```python
from build123d import *

# Parameters (mm, degrees)
SALIENTE_EXTRUIR1_DEPTH      = 35
SALIENTE_EXTRUIR1_DEPTH_BACK = 35
CORTAR_EXTRUIR1_DEPTH        = 3
CROQUIS4_R                   = 8
CORTAR_EXTRUIR2_DEPTH        = 3
CROQUIS5_R                   = 2.5
CORTAR_EXTRUIR3_DEPTH        = 10
CROQUIS6_W                   = 6
CROQUIS6_H                   = 10
CORTAR_EXTRUIR5_DEPTH        = 10
CROQUIS7_W                   = 2
CROQUIS7_H                   = 2
CORTAR_EXTRUIR6_DEPTH        = 5
CROQUIS8_R                   = 1
CORTAR_EXTRUIR7_DEPTH        = 2
CROQUIS9_W                   = 6
CROQUIS9_H                   = 10
CORTAR_EXTRUIR8_DEPTH        = 12
CORTAR_EXTRUIR9_DEPTH        = 5
CORTAR_EXTRUIR9_DEPTH_BACK   = 5
CROQUIS10_R                  = 1
CORTAR_EXTRUIR10_DEPTH       = 5
CORTAR_EXTRUIR10_DEPTH_BACK  = 5
CORTAR_EXTRUIR11_DEPTH       = 3
CORTAR_EXTRUIR11_DEPTH_BACK  = 3
CROQUIS15_R                  = 2.5
CORTAR_EXTRUIR12_DEPTH       = 15
CROQUIS14_W                  = 2
CROQUIS14_H                  = 10
CORTAR_EXTRUIR13_DEPTH       = 10


with BuildPart() as part:
    # Croquis1 → Saliente-Extruir1 (new, two sides: drawn at the far end of the back side and taken through both)
    with BuildSketch(Plane.XY.offset(-SALIENTE_EXTRUIR1_DEPTH_BACK)):
        with BuildLine():
            Line((-15, 0), (15, 0))
            ThreePointArc((15, 0), (0, -15), (-15, 0))
        make_face()
    extrude(amount=SALIENTE_EXTRUIR1_DEPTH + SALIENTE_EXTRUIR1_DEPTH_BACK)

    # Croquis3 → Cortar-Extruir1 (cut)
    with BuildSketch(Plane(origin=(0, 0, 0), x_dir=(1, 0, 0), z_dir=(0, 1, 0))):
        with BuildLine():
            Line((-8, 25), (-12.284525276, 15.598253186))
            ThreePointArc((-12.284525276, 15.598253186), (0, -3.5), (12.284525276, 15.598253186))
            Line((12.284525276, 15.598253186), (8, 25))
            ThreePointArc((8, 25), (13, 30), (8, 35))
            Line((8, 35), (-8, 35))
            ThreePointArc((-8, 35), (-13, 30), (-8, 25))
        make_face()
    extrude(amount=-CORTAR_EXTRUIR1_DEPTH, mode=Mode.SUBTRACT)

    # Croquis4 → Cortar-Extruir2 (cut)
    with BuildSketch(Plane(origin=(0, -3, 0), x_dir=(1, 0, 0), z_dir=(0, 1, 0))):
        with Locations(Location((0, 10, 0), (0, 0, 270))):
            Circle(CROQUIS4_R)
    extrude(amount=-CORTAR_EXTRUIR2_DEPTH, mode=Mode.SUBTRACT)

    # Croquis5 → Cortar-Extruir3 (cut)
    with BuildSketch(Plane(origin=(0, -6, 0), x_dir=(1, 0, 0), z_dir=(0, 1, 0))):
        with Locations(Location((0, 10, 0), (0, 0, 270))):
            Circle(CROQUIS5_R)
    extrude(amount=-CORTAR_EXTRUIR3_DEPTH, mode=Mode.SUBTRACT)

    # Croquis6 → Cortar-Extruir5 (cut)
    with BuildSketch(Plane(origin=(0, -3, 0), x_dir=(1, 0, 0), z_dir=(0, 1, 0))):
        with Locations((0, 30)):
            Rectangle(CROQUIS6_W, CROQUIS6_H)
    extrude(amount=-CORTAR_EXTRUIR5_DEPTH, mode=Mode.SUBTRACT)

    # Croquis7 → Cortar-Extruir6 (cut)
    with BuildSketch(Plane(origin=(0, -3, 0), x_dir=(1, 0, 0), z_dir=(0, 1, 0))):
        with Locations((-4, 30)):
            Rectangle(CROQUIS7_W, CROQUIS7_H)
        with Locations((4, 30)):
            Rectangle(CROQUIS7_W, CROQUIS7_H)
    extrude(amount=-CORTAR_EXTRUIR6_DEPTH, mode=Mode.SUBTRACT)

    # Croquis8 → Cortar-Extruir7 (cut)
    with BuildSketch(Plane(origin=(0, -3, 0), x_dir=(1, 0, 0), z_dir=(0, 1, 0))):
        with Locations(Location((-8, 30, 0), (0, 0, 270))):
            Circle(CROQUIS8_R)
        with Locations(Location((8, 30, 0), (0, 0, 270))):
            Circle(CROQUIS8_R)
    extrude(amount=-CORTAR_EXTRUIR7_DEPTH, mode=Mode.SUBTRACT)

    # Croquis9 → Cortar-Extruir8 (cut)
    with BuildSketch(Plane(origin=(0, -3, 0), x_dir=(1, 0, 0), z_dir=(0, 1, 0))):
        Rectangle(CROQUIS9_W, CROQUIS9_H)
    extrude(amount=-CORTAR_EXTRUIR8_DEPTH, mode=Mode.SUBTRACT)

    # Croquis10 → Cortar-Extruir9 (cut, two sides: drawn at the far end of the back side and taken through both)
    with BuildSketch(Plane(origin=(0, 0, 0), x_dir=(0, 0, -1), z_dir=(1, 0, 0)).offset(-CORTAR_EXTRUIR9_DEPTH_BACK)):
        with Locations((30, -8)):
            Circle(CROQUIS10_R)
    extrude(amount=CORTAR_EXTRUIR9_DEPTH + CORTAR_EXTRUIR9_DEPTH_BACK, mode=Mode.SUBTRACT)

    # Croquis11 → Cortar-Extruir10 (cut, two sides: drawn at the far end of the back side and taken through both)
    with BuildSketch(Plane(origin=(0, 0, 0), x_dir=(0, 0, -1), z_dir=(1, 0, 0)).offset(-CORTAR_EXTRUIR10_DEPTH_BACK)):
        with BuildLine():
            Line((-6, -15), (6, -15))
            Line((6, -15), (6, -14))
            Line((6, -14), (1, -14))
            Line((1, -14), (1, -8))
            ThreePointArc((1, -8), (0, -7), (-1, -8))
            Line((-1, -8), (-1, -14))
            Line((-1, -14), (-6, -14))
            Line((-6, -14), (-6, -15))
        make_face()
    extrude(amount=CORTAR_EXTRUIR10_DEPTH + CORTAR_EXTRUIR10_DEPTH_BACK, mode=Mode.SUBTRACT)

    # Croquis12 → Cortar-Extruir11 (cut, two sides: drawn at the far end of the back side and taken through both)
    with BuildSketch(Plane(origin=(0, 0, 0), x_dir=(0, 0, -1), z_dir=(1, 0, 0)).offset(-CORTAR_EXTRUIR11_DEPTH_BACK)):
        with BuildLine():
            Line((-3, -13), (-21.658767316, -9.861464952))
            ThreePointArc((-21.658767316, -9.861464952), (-27.635040051, -6.458030924), (-30, 0))
            Line((-30, 0), (-3, 0))
            Line((-3, 0), (-3, -13))
        make_face()
        Polygon((25, -8), (25, -3), (4, -3), (4, -13), align=None)
    extrude(amount=CORTAR_EXTRUIR11_DEPTH + CORTAR_EXTRUIR11_DEPTH_BACK, mode=Mode.SUBTRACT)

    # Croquis15 → Cortar-Extruir12 (cut)
    with BuildSketch(Plane(origin=(0, 0, 0), x_dir=(0, 0, -1), z_dir=(1, 0, 0))):
        with Locations((-20, 0)):
            Circle(CROQUIS15_R)
    extrude(amount=-CORTAR_EXTRUIR12_DEPTH, mode=Mode.SUBTRACT)

    # Croquis14 → Cortar-Extruir13 (cut)
    with BuildSketch(Plane(origin=(0, 0, 0), x_dir=(1, 0, 0), z_dir=(0, 1, 0))):
        with Locations((4, -20)):
            Rectangle(CROQUIS14_W, CROQUIS14_H)
        with Locations((-4, -20)):
            Rectangle(CROQUIS14_W, CROQUIS14_H)
    extrude(amount=-CORTAR_EXTRUIR13_DEPTH, mode=Mode.SUBTRACT)


solid = part.part
```
The model under review builds one solid part; all positions refer to its coordinate system, in mm. A direction names the side the tool comes from. Round coordinates to 2 decimals unless told otherwise and drop trailing zeros. Order: outer loops, then holes, each group sorted by start corner. A loop starts at its lowest first (then second) coordinate and runs counter-clockwise, first axis right, second up.
Item 1: Machinability: for faces 1 (the flat face through (-5, -11, 0)), 2 (the cylindrical face through (-9.9, -2.5, 20.1)), 3 (the flat face through (-5, -6, -10)), which of the approach directions +Z, -Z, +X, -X, +Y, -Y give a long, thin tool a straight path to every point of the face, cutting with its end or side? Answer none if there is none.
Working result:
face 1: -Y
face 2: -X, +Y
face 3: +Y
Item 2: Add section B-B, the plane x = -11.5. State the section outline as (y, z) points.
Working result:
outline: (-9.63, -35) - (0, -35) - (0, -33.57) - (-3, -33.57) - (-3, -26.43) - (0, -26.43) - (0, -17.32) - (-3, -17.32) - (-3, -2.93) - (0, -2.93) - (0, 17.5) arc R2.5 cw to (0, 22.5) - (0, 35) - (-9.63, 35) - close
Item 3: Draft analysis for pull direction Z (two halves, no side actions). For faces 4 (the cylindrical face through (12.024, -1.479, -3.862)), 5 (the flat face through (5, 0, 13)), state which applies: released by +Z, released by -Z, zero draft, split by the parting line, or undercut.
Working result:
face 4: undercut
face 5: zero draft
Item 4: To check wall thickness, follow probe 1 along Z at (x, y) = (0, -13.25); probe 2 along Z at (x, y) = (0, -14.05); probe 3 along X at (y, z) = (-3.8, -30). State the ranges of each line that lie inside material, in increasing order.
Working result:
probe 1: z = -35 to -12.5, -7.5 to -5, 5 to 35
probe 2: z = -35 to -12.5, -7.5 to -6, 6 to 35
probe 3: x = -14.51 to -9, -7 to -5, 5 to 7, 9 to 14.51
Item 5: Add section A-A, the plane z = -10. State the section outline as (x, y) points, and give its area (3 significant figures).
Working result:
outline: (-15, 0) arc R15 ccw to (-2.5, -14.79) - (-2.5, -11.57) - (-3, -11.57) - (-3, -6) - (-8, -6) - (-8, -3) - (-13.5, -3) - (-13.5, 0) - close; (2.5, -14.79) arc R15 ccw to (15, 0) - (13.5, 0) - (13.5, -3) - (8, -3) - (8, -6) - (3, -6) - (3, -11.57) - (2.5, -11.57) - close
area: 174 mm2
Item 6: Add section D-D, the plane z = 0. State the section outline as (x, y) points, and give its area (3 significant figures).
Working result:
outline: (-15, 0) arc R15 ccw to (-5, -14.14) - (-5, -7) - (-3, -7) - (-3, -3) - (-9.07, -3) - (-9.07, 0) - close; (3, -7) - (5, -7) - (5, -14.14) arc R15 ccw to (15, 0) - (9.07, 0) - (9.07, -3) - (3, -3) - close
area: 198 mm2
Item 7: Add section C-C, the plane z = -30. State the section outline as (x, y) points, and give its area (3 significant figures).
Working result:
outline: (-15, 0) arc R15 ccw to (15, 0) - (13, 0) - (13, -3) - (9, -3) - (9, -5) - (7, -5) - (7, -3) - (5, -3) - (5, -9) - (3, -9) - (3, -13) - (-3, -13) - (-3, -9) - (-5, -9) - (-5, -3) - (-7, -3) - (-7, -5) - (-9, -5) - (-9, -3) - (-13, -3) - (-13, 0) - close
area: 183 mm2
Item 8: For pin 1 (3 mm diameter, centred on x = 0.5, z = -28.5, fed in from +Y); pin 2 (5.5 mm diameter, centred on x = -6.5, z = -7, fed in from +Y); pin 3 (1 mm diameter, centred on x = 4, z = 20.5, fed in from +Y), all flat-tipped, find the tip position at first contact; note any pin that passes through.
Working result:
pin 1: stops at y = -13
pin 2: stops at y = -3
pin 3: stops at y = -10
